Build history of the part. All positions in model axes, mm. A direction names the side the tool comes from. Give positions to 0.01 mm unless a question says otherwise; leave off trailing zeros. Loops run counter-clockwise (first coordinate to the right, second up) from the corner with the lowest first, then second, coordinate; pieces in that order, holes last. Notation, with made-up numbers: M 62,-17 L 94,-17 A16 ccw 94,-4 Z; hole C 60.25,26.5 d3. An arc over 180 degrees is marked long. Answer as a JSON object with one key per item and string values. Group by question number.
1. Drop a flat-ended pin along its axis: pin 1 Ø5 at (x, y) = (-22, 26.5) entering from +Z. Give the stop position or say it passes through.
2. 3-axis set-ups, long thin cutter, end or side, ignore diameter. For faces 1 (the face through (-1, -30.6, 10)), 2 (the face through (-54, -1, 7)): which of +Z, -Z, +X, -X, +Y, -Y reach the whole face in a straight line?
3. Slice it at B-B (y = -37). List the corners of the cut face in (x, z).
4. Mould opens along Y. For faces 3 (the face through (-1, 1, 0)), 4 (the face through (-1, -44, 7)), 5 (the face through (-1, 44, 7)), 6 (the face through (45.254, -38.339, 6.902)) say: released by +Y, released by -Y, zero draft, split by the parting line, or undercut.
5. Drill centre lines: line 1 along Y through (x, z) = (47, 5); line 2 along Y through (x, z) = (32.5, 12); line 3 along X through (y, z) = (23, 11.5). Where is each one in solid material? Low to high. Write a range as [from, to].
6. Slice it at C-C (z = 9). List the corners of the cut face in (x, y), then the cut area to 3 significant figures.
7. Slice it at A-A (x = -47). List the corners of the cut face in (y, z), then the cut area to 3 significant figures.
8. Slice it at D-D (x = 8). List the corners of the cut face in (y, z), then the cut area to 3 significant figures.
from build123d import *

# Parameters (mm, degrees)
SKETCH2_W                   = 108
SKETCH2_H                   = 88
FIXTURE_FLOOR_DEPTH         = 6
ENCLOSURE_NEST_START        = 6
SKETCH3_W                   = 108
SKETCH3_H                   = 88
SKETCH3_W_2                 = 81.2
SKETCH3_H_2                 = 61.2
ENCLOSURE_NEST_DEPTH        = 8
SKETCH4_R                   = 2.2
BENCH_MOUNT_CLEARANCE_DEPTH = 14
SKETCH5_R                   = 2.2
CUT_EXTRUDE2_DEPTH          = 14
SKETCH6_R                   = 2.2
CUT_EXTRUDE3_DEPTH          = 14
SKETCH7_R                   = 2.2
CUT_EXTRUDE4_DEPTH          = 14


with BuildPart() as part:
    # Sketch2 → Fixture_floor (new body)
    with BuildSketch(Plane.XY):
        Rectangle(SKETCH2_W, SKETCH2_H)
    extrude(amount=FIXTURE_FLOOR_DEPTH)

    # Sketch3 → Enclosure_nest (add)
    with BuildSketch(Plane.XY.offset(ENCLOSURE_NEST_START)):
        Rectangle(SKETCH3_W, SKETCH3_H)
        Rectangle(SKETCH3_W_2, SKETCH3_H_2, mode=Mode.SUBTRACT)
    extrude(amount=ENCLOSURE_NEST_DEPTH)

    # Sketch4 → Bench_mount_clearance (cut)
    with BuildSketch(Plane.XY):
        with Locations((-47, -37)):
            Circle(SKETCH4_R)
    extrude(amount=BENCH_MOUNT_CLEARANCE_DEPTH, mode=Mode.SUBTRACT)

    # Sketch5 → Cut-Extrude2 (cut)
    with BuildSketch(Plane.XY):
        with Locations((-47, 37)):
            Circle(SKETCH5_R)
    extrude(amount=CUT_EXTRUDE2_DEPTH, mode=Mode.SUBTRACT)

    # Sketch6 → Cut-Extrude3 (cut)
    with BuildSketch(Plane.XY):
        with Locations((47, -37)):
            Circle(SKETCH6_R)
    extrude(amount=CUT_EXTRUDE3_DEPTH, mode=Mode.SUBTRACT)

    # Sketch7 → Cut-Extrude4 (cut)
    with BuildSketch(Plane.XY):
        with Locations((47, 37)):
            Circle(SKETCH7_R)
    extrude(amount=CUT_EXTRUDE4_DEPTH, mode=Mode.SUBTRACT)


solid = part.part
Established:
{
 "1": {"pin 1": "stops at z = 6"},
 "2": {"face 1": "+Z", "face 2": "+Z, -Z, -X, +Y, -Y"},
 "3": {"outline": "M -54,0 L -49.2,0 L -49.2,14 L -54,14 Z; M -44.8,0 L 44.8,0 L 44.8,14 L -44.8,14 Z; M 49.2,0 L 54,0 L 54,14 L 49.2,14 Z"},
 "4": {"face 3": "zero draft", "face 4": "released by -Y", "face 5": "released by +Y", "face 6": "undercut"},
 "5": {"line 1": "y = [-44, -39.2], [-34.8, 34.8], [39.2, 44]", "line 2": "y = [-44, -30.6], [30.6, 44]", "line 3": "x = [-54, -40.6], [40.6, 54]"},
 "6": {"outline": "M -54,-44 L 54,-44 L 54,44 L -54,44 Z; hole C -47,-37 d4.4; hole C -47,37 d4.4; hole M -40.6,-30.6 L 40.6,-30.6 L 40.6,30.6 L -40.6,30.6 Z; hole C 47,-37 d4.4; hole C 47,37 d4.4", "area": "4,470 mm^2"},
 "7": {"outline": "M -44,0 L -39.2,0 L -39.2,14 L -44,14 Z; M -34.8,0 L 34.8,0 L 34.8,14 L -34.8,14 Z; M 39.2,0 L 44,0 L 44,14 L 39.2,14 Z", "area": "1,110 mm^2"},
 "8": {"outline": "M -44,0 L 44,0 L 44,14 L 30.6,14 L 30.6,6 L -30.6,6 L -30.6,14 L -44,14 Z", "area": "742 mm^2"}
}
